Design review of the part built by this model. Coordinates are the model's own, in mm. Give positions to 0.01 mm unless a question says otherwise; leave off trailing zeros. Loops run counter-clockwise (first coordinate to the right, second up) from the corner with the lowest first, then second, coordinate; pieces in that order, holes last. Notation, with made-up numbers: M 56.25,11.25 L 108.25,11.25 A35 cw 108.25,45.25 Z; hole C 15.25,39.25 d11. An arc over 180 degrees is marked long. Use a Markdown table: item, result. Add a question column.
(1) For probe 1 along X at (y, z) = (-4.75, 0.25); probe 2 along Y at (x, z) = (28.5, 1.75); probe 3 along Z at (x, y) = (15, -2.5), list the stretches that pass through material, from the lowest coordinate up.
(2) Insertion check: pin 1 Ø3 at (x, y) = (8, 2) entering from +Z; pin 2 Ø5 at (x, y) = (35.5, -1) entering from -Z; pin 3 Ø1.5 at (x, z) = (31, -0.5) entering from -Y. Each pin has a flat end and moves straight along its axis. Give the tip position at first contact, or say it passes through.
(3) Add section A-A, the plane x = 31. Give the boundary of the cut face in (y, z), then the cut area to 3 significant figures.
```python
from build123d import *

# Parameters (mm, degrees)
BASEHEAD_DEPTH   = 5.3
SKETCH5_R        = 4
BASEBODY_DEPTH   = 65
CHAMFER1_SIZE    = 0.4
LPATTERN10_COUNT = 27
LPATTERN10_PITCH = 0.8118


with BuildPart() as part:
    # Sketch2 → BaseHead (new body)
    with BuildSketch(Plane(origin=(0, 0, 0), x_dir=(0, 0, -1), z_dir=(1, 0, 0))):
        Polygon((0, -7.505553499), (6.5, -3.75277675), (6.5, 3.75277675), (0, 7.505553499), (-6.5, 3.75277675), (-6.5, -3.75277675), align=None)
    extrude(amount=BASEHEAD_DEPTH)

    # Sketch3 → BearingFace (revolve, cut)
    with BuildSketch(Plane.XY, mode=Mode.PRIVATE) as bearingface_sk:
        Polygon((5.3, 7.505553499), (5.3, 5.735), (4.7, 6.335), (4.7, 7.505553499), align=None)
    revolve(bearingface_sk.sketch.rotate(Axis((-0.957090588, 0, 0), (1, 0, 0)), 90), axis=Axis((-0.957090588, 0, 0), (1, 0, 0)), mode=Mode.SUBTRACT)

    # Sketch4 → HeadChamfer (revolve, cut)
    with BuildSketch(Plane.XY):
        Polygon((0, 7.505553499), (0.365991543, 7.505553499), (0, 6.5), align=None)
    revolve(axis=Axis((-0.493528746, 0, 0), (1, 0, 0)), mode=Mode.SUBTRACT)

    # Sketch5 → BaseBody (add)
    with BuildSketch(Plane(origin=(5.3, 0, 0), x_dir=(0, 0, -1), z_dir=(1, 0, 0))):
        with Locations(Location((0, 0, 0), (0, 0, 180))):
            Circle(SKETCH5_R)
    extrude(amount=BASEBODY_DEPTH)

    # Chamfer1
    chamfer1_edges = [part.edges().sort_by_distance(p)[0] for p in [
        (70.3, 0, -4),
    ]]
    chamfer(chamfer1_edges, length=CHAMFER1_SIZE)

    # Sketch6 → Cut-Revolve10 (revolve, cut)
    with BuildSketch(Plane.XY, mode=Mode.PRIVATE) as cut_revolve10_sk:
        Polygon((69.2235, 4.6765), (69.9, 4.6765), (69.9, 4), (69.56175, 3.414133814), (69.2235, 4), align=None)
    cut_revolve10 = revolve(cut_revolve10_sk.sketch.rotate(Axis((70.3, 0, 0), (-1, 0, 0)), 90), axis=Axis((70.3, 0, 0), (-1, 0, 0)), mode=Mode.SUBTRACT)

    # LPattern10: Cut-Revolve10 ×27
    with Locations(*[(-i * LPATTERN10_PITCH, 0, 0) for i in range(1, LPATTERN10_COUNT)]):
        add(cut_revolve10, mode=Mode.SUBTRACT)


solid = part.part
```
Established:
| question | item | result |
|---|---|---|
| 1 | probe 1 | 0 to 5.3 |
| 1 | probe 2 | -3.6 to 3.6 |
| 1 | probe 3 | -3.12 to 3.12 |
| 2 | pin 1 | z = 3.97 |
| 2 | pin 2 | z = -4 |
| 2 | pin 3 | y = -4 |
| 3 | outline | C 0,0 d8 |
| 3 | area | 50.3 mm^2 |
